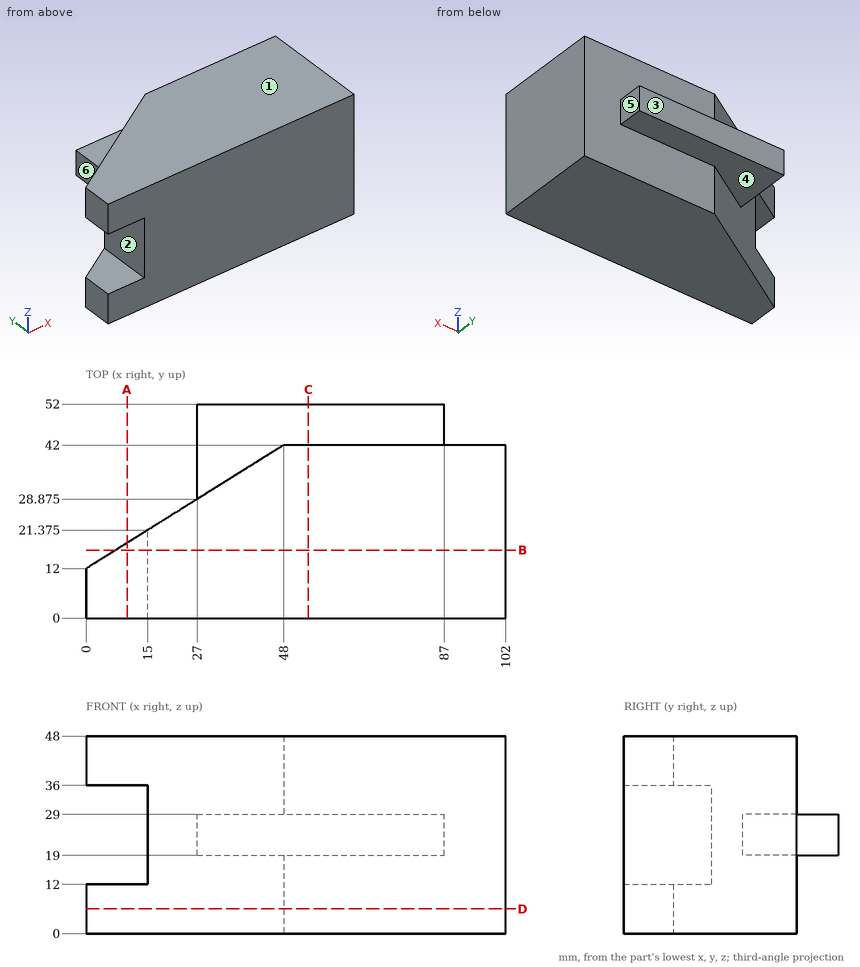
Verification items for this drawing (mm, ordinates from the low corner). A direction names the side the tool comes from. Coordinates: 2 decimals unless noted, no trailing zeros. Loops run counter-clockwise (first coordinate to the right, second up) from the corner with the lowest first, then second, coordinate; pieces in that order, holes last. Notation, with made-up numbers: (87.5, 69) - (112.5, 69) arc R14 ccw to (112.5, 79) - close; hole circle Ø2 at (77, 69). An arc over 180 degrees is marked (long way). Use one line per item in the form item = value. Start each with the question number.
Item 1: Thickness scan on probe 1 along X at (y, z) = (10.5, 24.5); probe 2 along Y at (x, z) = (52, 13.5); probe 3 along Z at (x, y) = (82, 44.5). Record the ranges inside material, lowest first.
Item 2: Mould release check, pull along Z, two halves, no side actions. Record for the marked faces 1, 2 and 3: +Z half, -Z half, draft (parallel to the pull), parting line (faces both ways), or undercut.
Item 3: Section check C-C, the plane x = 54. Enter the section's corners in (y, z).
Item 4: Section check B-B, the plane y = 16.5. Enter the section's corners in (x, z), and give its area (3 significant figures).
Item 5: Section check D-D, the plane z = 6. Enter the section's corners in (x, y).
Item 6: Gauge pin test, flat ends, axial feed: pin 1 (2 mm diameter, centred on y = 22.5, z = 19, fed in from -X); pin 2 (11 mm diameter, centred on y = 36, z = 24, fed in from -X); pin 3 (6 mm diameter, centred on x = 18.5, z = 6.5, fed in from +Y). Record the tip position at first contact, or that the pin passes through.
Item 7: Tool access check on the marked faces 4, 5 and 6. Record the directions out of +Z, -Z, +X, -X, +Y, -Y that give a thin tool (end or side, any length) a straight path to the whole face; none if there is none.
Item 8: Section check A-A, the plane x = 10. Enter the section's corners in (y, z), and give its area (3 significant figures).
Computed:
q1.probe_1 = 15 to 102
q1.probe_2 = 0 to 42
q1.probe_3 = 19 to 29
q2.face_1 = +Z half
q2.face_2 = undercut
q2.face_3 = draft
q3.outline = (0, 0) - (42, 0) - (42, 19) - (52, 19) - (52, 29) - (42, 29) - (42, 48) - (0, 48) - close
q4.outline = (7.2, 0) - (102, 0) - (102, 48) - (7.2, 48) - (7.2, 36) - (15, 36) - (15, 12) - (7.2, 12) - close
q4.area = 4,360 mm2
q5.outline = (0, 0) - (102, 0) - (102, 42) - (48, 42) - (0, 12) - close
q6.pin_1 = 15.2
q6.pin_2 = 27
q6.pin_3 = 25.44
q7.face_4 = -Z, -X, +Y
q7.face_5 = +Z, -Z, +X, +Y
q7.face_6 = +Z, -Z, -X, +Y
q8.outline = (0, 0) - (18.25, 0) - (18.25, 12) - (0, 12) - close; (0, 36) - (18.25, 36) - (18.25, 48) - (0, 48) - close
q8.area = 438 mm2
